Source: CAD feature listing. Evaluate the final solid. Frame: model axes, mm. Face numbers are marked on the shaded views. A direction names the side the tool comes from. Give positions to 0.01 mm unless a question says otherwise; leave off trailing zeros. Loops run counter-clockwise (first coordinate to the right, second up) from the corner with the lowest first, then second, coordinate; pieces in that order, holes last. Notation, with made-up numbers: M -32.75,-10.75 L -4.75,-10.75 A13 cw -4.75,0.25 Z; hole C -11,-9 d10. An arc over 180 degrees is marked long. Answer in a Markdown table with one row per item.
```python
from build123d import *

# Parameters (mm, degrees)
SALIENTE_EXTRUIR1_DEPTH = 10


with BuildPart() as part:
    # Croquis1 → Saliente-Extruir1 (new body)
    with BuildSketch(Plane.XY):
        with BuildLine():
            Line((1.5, -23.5), (6, -23.5))
            ThreePointArc((6, -23.5), (6.707106781, -23.207106781), (7, -22.5))
            Line((7, -22.5), (7, -15.5))
            ThreePointArc((7, -15.5), (6.707106781, -14.792893219), (6, -14.5))
            Line((6, -14.5), (4.934593139, -14.5))
            Line((4.934593139, -14.5), (4.934593139, -7.41826154))
            ThreePointArc((4.934593139, -7.41826154), (5.033290189, -6.985072213), (5.309899124, -6.637391904))
            ThreePointArc((5.309899124, -6.637391904), (0, 8.5), (-5.309899124, -6.637391904))
            ThreePointArc((-5.309899124, -6.637391904), (-5.033290189, -6.985072213), (-4.934593139, -7.41826154))
            Line((-4.934593139, -7.41826154), (-4.934593139, -14.5))
            Line((-4.934593139, -14.5), (-6, -14.5))
            ThreePointArc((-6, -14.5), (-6.707106781, -14.792893219), (-7, -15.5))
            Line((-7, -15.5), (-7, -22.5))
            ThreePointArc((-7, -22.5), (-6.707106781, -23.207106781), (-6, -23.5))
            Line((-6, -23.5), (-1.5, -23.5))
            ThreePointArc((-1.5, -23.5), (-0.792893219, -23.207106781), (-0.5, -22.5))
            Line((-0.5, -22.5), (-0.5, -5.291502622))
            ThreePointArc((-0.5, -5.291502622), (-0.702275965, -4.688479933), (-1.227272727, -4.329411236))
            ThreePointArc((-1.227272727, -4.329411236), (0, 4.5), (1.227272727, -4.329411236))
            ThreePointArc((1.227272727, -4.329411236), (0.702275965, -4.688479933), (0.5, -5.291502622))
            Line((0.5, -5.291502622), (0.5, -22.5))
            ThreePointArc((0.5, -22.5), (0.792893219, -23.207106781), (1.5, -23.5))
        make_face()
    extrude(amount=SALIENTE_EXTRUIR1_DEPTH)


solid = part.part
```
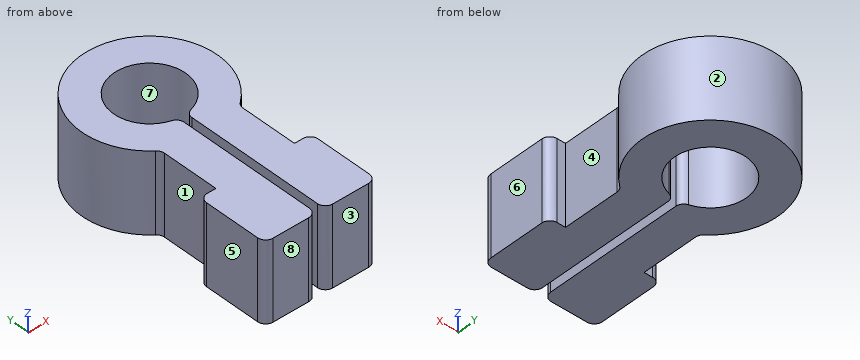
1) Set-up query: the marked faces 1, 2, 3, 4 and 5. Return all of +Z, -Z, +X, -X, +Y, -Y with unobstructed straight access to the full face (end or side cutting, diameter ignored); none if empty.
Reply:
| item | result |
|---|---|
| face 1 | +Z, -Z, -X |
| face 2 | +Z, -Z |
| face 3 | +Z, -Z, +X, -X, -Y |
| face 4 | +Z, -Z, +X |
| face 5 | +Z, -Z, -X, -Y |
2) Pin query (flat end, axial travel): pin 1 Ø6 at (y, z) = (-14.5, 7) entering from -X; pin 2 Ø4 at (y, z) = (-5.5, 7.5) entering from +X; pin 3 Ø0.9 at (x, z) = (5.5, 3) entering from +Y; pin 4 Ø7 at (x, y) = (0, 0) entering from +Z. Return the tip coordinate at first contact, or that it passes through.
Reply:
| item | result |
|---|---|
| pin 1 | stops at x = -7 |
| pin 2 | stops at x = 7.75 |
| pin 3 | stops at y = 6.84 |
| pin 4 | passes through |
3) Section A-A, the plane y = -14. Return loops of the section in (x, z).
Reply:
| item | result |
|---|---|
| outline | M -4.93,0 L -0.5,0 L -0.5,10 L -4.93,10 Z; M 0.5,0 L 4.93,0 L 4.93,10 L 0.5,10 Z |
4) Section C-C, the plane z = 3.75. Return loops of the section in (x, y).
Reply:
| item | result |
|---|---|
| outline | M -7,-22.5 A1 ccw -6,-23.5 L -1.5,-23.5 A1 ccw -0.5,-22.5 L -0.5,-5.29 A1 ccw -1.23,-4.33 A4.5 cw long 1.23,-4.33 A1 ccw 0.5,-5.29 L 0.5,-22.5 A1 ccw 1.5,-23.5 L 6,-23.5 A1 ccw 7,-22.5 L 7,-15.5 A1 ccw 6,-14.5 L 4.93,-14.5 L 4.93,-7.42 A1 cw 5.31,-6.64 A8.5 ccw long -5.31,-6.64 A1 cw -4.93,-7.42 L -4.93,-14.5 L -6,-14.5 A1 ccw -7,-15.5 Z |
5) Pull-direction query (Y, two-part tool) for the marked faces 6, 7 and 8; classes: released by +Y, released by -Y, zero draft, split by the parting line, or undercut.
Reply:
| item | result |
|---|---|
| face 6 | zero draft |
| face 7 | undercut |
| face 8 | released by -Y |
6) Section B-B, the plane x = 2.25. Return loops of the section in (y, z).
Reply:
| item | result |
|---|---|
| outline | M -23.5,0 L -3.9,0 L -3.9,10 L -23.5,10 Z; M 3.9,0 L 8.2,0 L 8.2,10 L 3.9,10 Z |
7) Material intervals for L1, parallel to X at y = -12.5, z = 9.25; L2, parallel to X at y = 0, z = 7.5; L3, parallel to Y at x = 0, z = 8.25, sorted ascending.
Reply:
| item | result |
|---|---|
| L1 | x = -4.93 to -0.5, 0.5 to 4.93 |
| L2 | x = -8.5 to -4.5, 4.5 to 8.5 |
| L3 | y = 4.5 to 8.5 |
8) Section D-D, the plane x = 0. Return loops of the section in (y, z).
Reply:
| item | result |
|---|---|
| outline | M 4.5,0 L 8.5,0 L 8.5,10 L 4.5,10 Z |
